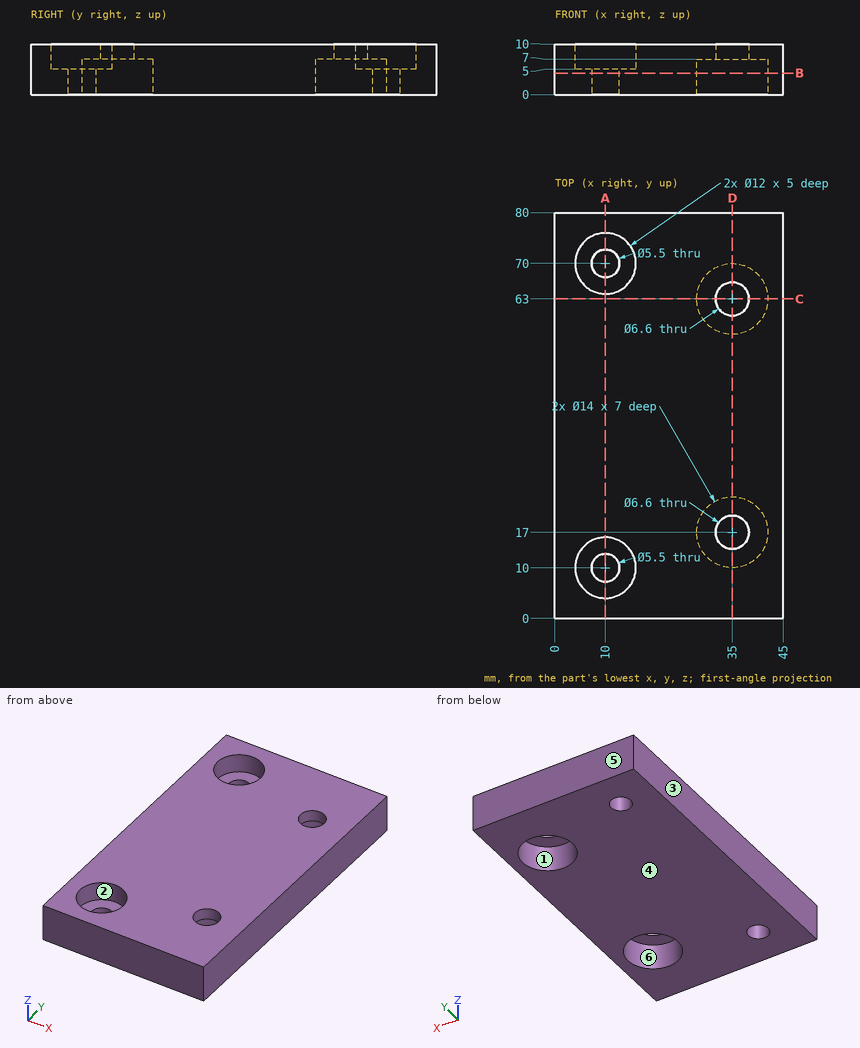
Source: three-view drawing plus pictorial views. Frame: mm from the lowest corner of the part. A direction names the side the tool comes from. Coordinates: 2 decimals unless noted, no trailing zeros. Write each loop counter-clockwise with the first axis right and the second up, starting at its lowest first coordinate (ties: lowest second). Pieces come first, ordered by that corner, then holes. Notation, with made-up numbers: (-18, -35) -> (23, -35) arc R19 cw to (23, -29) -> close; hole circle Ø2 at (41, -8.75). An arc over 180 degrees is marked (long way). Write each question's results on one line, items separated by ' | '.
Item 1: Mould query, pull axis Y, two halves, no side actions, for the marked faces 4, 5 and 6. Classes: +Y half, -Y half, draft (parallel to the pull), parting line (faces both ways), or undercut.
Conclusion:
face 4: draft | face 5: +Y half | face 6: undercut
Item 2: Section query A-A on x = 10. Return loops of the section in (y, z), plus the area to 3 significant figures.
Conclusion:
outline: (0, 0) -> (7.25, 0) -> (7.25, 5) -> (4, 5) -> (4, 10) -> (0, 10) -> close; (12.75, 0) -> (67.25, 0) -> (67.25, 5) -> (64, 5) -> (64, 10) -> (16, 10) -> (16, 5) -> (12.75, 5) -> close; (72.75, 0) -> (80, 0) -> (80, 10) -> (76, 10) -> (76, 5) -> (72.75, 5) -> close | area: 625 mm^2
Item 3: Pin query (flat end, axial travel): pin 1 Ø7 at (x, y) = (37, 63) entering from -Z; pin 2 Ø3.5 at (x, y) = (9.5, 71) entering from +Z. Return the tip coordinate at first contact, or that it passes through.
Conclusion:
pin 1: stops at z = 7 | pin 2: stops at z = 5
Item 4: Section query C-C on y = 63. Return loops of the section in (x, z).
Conclusion:
outline: (0, 0) -> (28, 0) -> (28, 7) -> (31.7, 7) -> (31.7, 10) -> (0, 10) -> close; (38.3, 7) -> (42, 7) -> (42, 0) -> (45, 0) -> (45, 10) -> (38.3, 10) -> close
Item 5: Section query B-B on z = 4.25. Return loops of the section in (x, y).
Conclusion:
outline: (0, 0) -> (45, 0) -> (45, 80) -> (0, 80) -> close; hole circle Ø5.5 at (10, 10); hole circle Ø5.5 at (10, 70); hole circle Ø14 at (35, 17); hole circle Ø14 at (35, 63)
Item 6: Material intervals for probe 1 along Y at (x, z) = (35, 2.5); probe 2 along Y at (x, z) = (35, 7.85); probe 3 along X at (y, z) = (12, 2.5), sorted ascending.
Conclusion:
probe 1: y = 0 to 10, 24 to 56, 70 to 80 | probe 2: y = 0 to 13.7, 20.3 to 59.7, 66.3 to 80 | probe 3: x = 0 to 8.11, 11.89 to 30.1, 39.9 to 45
Item 7: Set-up query: the marked faces 1, 2 and 3. Return all of +Z, -Z, +X, -X, +Y, -Y with unobstructed straight access to the full face (end or side cutting, diameter ignored); none if empty.
Conclusion:
face 1: -Z | face 2: +Z | face 3: +Z, -Z, -X, +Y, -Y
Item 8: Section query D-D on x = 35. Return loops of the section in (y, z), plus the area to 3 significant figures.
Conclusion:
outline: (0, 0) -> (10, 0) -> (10, 7) -> (13.7, 7) -> (13.7, 10) -> (0, 10) -> close; (20.3, 7) -> (24, 7) -> (24, 0) -> (56, 0) -> (56, 7) -> (59.7, 7) -> (59.7, 10) -> (20.3, 10) -> close; (66.3, 7) -> (70, 7) -> (70, 0) -> (80, 0) -> (80, 10) -> (66.3, 10) -> close | area: 564 mm^2
